Check sheet for the modelled part. Datum: model origin and axes. Units: mm. A direction names the side the tool comes from. Give positions to 0.01 mm unless a question says otherwise; leave off trailing zeros. Loops run counter-clockwise (first coordinate to the right, second up) from the corner with the lowest first, then second, coordinate; pieces in that order, holes last. Notation, with made-up numbers: (79.5, 61) -> (131.5, 61) arc R27 ccw to (131.5, 84) -> close; hole circle Ø6 at (-11, -15). An arc over 180 degrees is marked (long way). Write each question's results on one line, items separated by ' | '. Start each with the question number.
1. Cross-section at D-D on z = 17.75. Record the boundary of the cut face in (x, y).
2. Cross-section at C-C on z = 3.5. Record the boundary of the cut face in (x, y).
3. Cross-section at A-A on y = -9. Record the boundary of the cut face in (x, z).
4. Tool access check on faces 5 (the face through (9.05, -19.75, 23.12)), 6 (the face through (28.61, -1.75, 21.49)), 7 (the face through (9.05, 1.48, 23.12)). Record the directions out of +Z, -Z, +X, -X, +Y, -Y that give a thin tool (end or side, any length) a straight path to the whole face; none if there is none.
5. Gauge pin test, flat ends, axial feed: pin 1 Ø4 at (y, z) = (-10, 12) entering from +X; pin 2 Ø12 at (y, z) = (-33, 4) entering from +X; pin 3 Ø8 at (y, z) = (-16, 5) entering from +X. Record the tip position at first contact, or that the pin passes through.
6. Material ranges on L1, parallel to Y at x = 3.5, z = 9.25; L2, parallel to Y at x = 11, z = 17; L3, parallel to Z at x = 27.5, y = -1.55, recorded low to high. Write a range as from..to.
7. Mould release check, pull along Z, two halves, no side actions. Record for faces 1 (the face through (16, -7, 15.5)), 2 (the face through (0, -1, 13)), 3 (the face through (29.797, -0.986, 1.141)), 4 (the face through (22.5, -7, 13)): +Z half, -Z half, draft (parallel to the pull), parting line (faces both ways), or undercut.
8. Cross-section at B-B on x = 15.5. Record the boundary of the cut face in (y, z).
from build123d import *

# Parameters (mm, degrees)
F1_DEPTH       = 2
F2_D           = 3
F2_CSINK_D     = 6
F2_CSINK_ANGLE = 90
F3_R           = 12
F4_DEPTH       = 3
F5_DEPTH       = 38
F6_R           = 10
F6_W           = 14
F6_H           = 5
F7_DEPTH       = 20


with BuildPart() as f1:
    # F0 (on Front) → F1 (new body)
    with BuildSketch(Plane.XZ):
        with BuildLine():
            ThreePointArc((0, 4), (1.1715728753, 1.1715728753), (4, 0))
            Line((4, 0), (27, 0))
            ThreePointArc((27, 0), (29.8284271247, 1.1715728753), (31, 4))
            Line((31, 4), (31, 22))
            ThreePointArc((31, 22), (29.8284271247, 24.8284271247), (27, 26))
            Line((27, 26), (4, 26))
            ThreePointArc((4, 26), (1.1715728753, 24.8284271247), (0, 22))
            Line((0, 22), (0, 4))
        make_face()
    extrude(amount=F1_DEPTH)

    # F2 (through all)
    with Locations(Plane(origin=(0, 0, 0), x_dir=(1, 0, 0), z_dir=(0, 1, 0))):
        with Locations((27.5, -22.5), (3.5, -3.5)):
            CounterSinkHole(F2_D / 2, F2_CSINK_D / 2, counter_sink_angle=F2_CSINK_ANGLE)

    # F3 (on face) → F4 (join)
    with BuildSketch(Plane(origin=(0, 0, 0), x_dir=(-1, 0, 0), z_dir=(0, 1, 0))):
        with Locations((-15.5, 13)):
            Circle(F3_R)
    extrude(amount=F4_DEPTH)

    # F3 (on face) → F5 (join)
    with BuildSketch(Plane(origin=(0, 0, 0), x_dir=(-1, 0, 0), z_dir=(0, 1, 0))):
        with Locations((-15.5, 13)):
            Circle(F3_R)
    extrude(amount=-F5_DEPTH)

    # F6 (on face) → F7 (cut)
    with BuildSketch(Plane(origin=(0, 3, 0), x_dir=(-1, 0, 0), z_dir=(0, 1, 0))):
        with Locations((-15.5, 13)):
            Circle(F6_R)
        with Locations((-15.5, 13)):
            Rectangle(F6_W, F6_H, mode=Mode.SUBTRACT)
    extrude(amount=-F7_DEPTH, mode=Mode.SUBTRACT)


solid = f1.part
Geometry says:
1) outline: (0, -2) -> (4.48, -2) -> (4.48, -38) -> (26.52, -38) -> (26.52, -2) -> (31, -2) -> (31, 0) -> (26.52, 0) -> (26.52, 3) -> (24.3, 3) -> (24.3, -17) -> (6.7, -17) -> (6.7, 3) -> (4.48, 3) -> (4.48, 0) -> (0, 0) -> close
2) outline: (0.03, -2) -> (2, -2) -> (2, -1.5) -> (0.5, 0) -> (0.03, 0) -> close; (5, -2) -> (8.17, -2) -> (8.17, -38) -> (22.83, -38) -> (22.83, -2) -> (30.97, -2) -> (30.97, 0) -> (22.83, 0) -> (22.83, 3) -> (18.62, 3) -> (18.62, -17) -> (12.38, -17) -> (12.38, 3) -> (8.17, 3) -> (8.17, 0) -> (6.5, 0) -> (5, -1.5) -> close
3) outline: circle Ø24 at (15.5, 13); (8.5, 10.5) -> (22.5, 10.5) -> (22.5, 15.5) -> (8.5, 15.5) -> close; hole circle Ø20 at (15.5, 13)
4) face 5: -Y | face 6: +Y, -Y | face 7: +Y
5) pin 1: x = 27.5 | pin 2: x = 27.12 | pin 3: x = 26.81
6) L1: -2..0 | L2: -38..-17 | L3: 0.03..21, 24..25.97
7) face 1: undercut | face 2: draft | face 3: -Z half | face 4: undercut
8) outline: (-38, 1) -> (-2, 1) -> (-2, 0) -> (0, 0) -> (0, 1) -> (3, 1) -> (3, 3) -> (-17, 3) -> (-17, 10.5) -> (3, 10.5) -> (3, 15.5) -> (-17, 15.5) -> (-17, 23) -> (3, 23) -> (3, 25) -> (0, 25) -> (0, 26) -> (-2, 26) -> (-2, 25) -> (-38, 25) -> close
